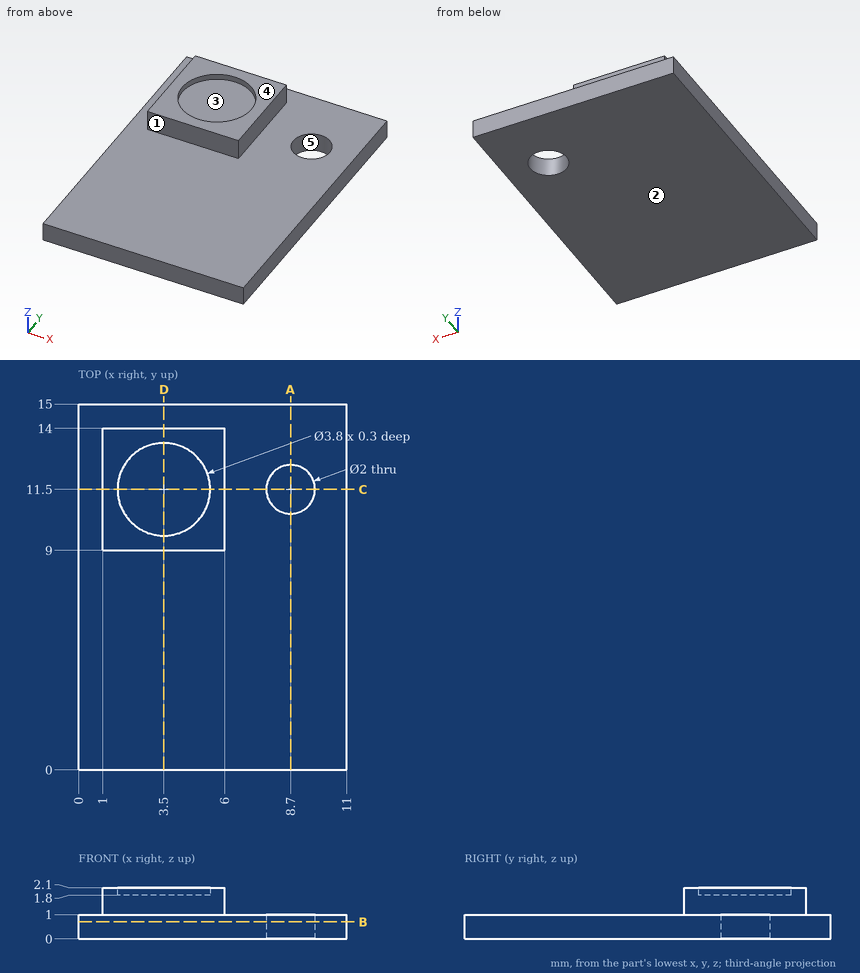
Could you check a few things on this drawing? It's one solid part, dimensions in mm from its lowest x, y, z. A direction names the side the tool comes from. Give positions to 0.01 mm unless a question says otherwise; leave off trailing zeros. Order: outer loops, then holes, each group sorted by start corner. A loop starts at its lowest first (then second) coordinate and runs counter-clockwise, first axis right, second up. Notation, with made-up numbers: M 72,80 L 83,80 A35 cw 83,116 Z; hole C 89.5,-22.75 d11. An arc over 180 degrees is marked long. Use one line per item in the form item = value.
Item 1: Will these pins go through, and if not, where does the flat tip stop? pin 1 Ø3.5 at (x, y) = (3.5, 11.5) entering from +Z; pin 2 Ø2.5 at (x, y) = (8.7, 11.5) entering from +Z; pin 3 Ø0.9 at (y, z) = (11, 1.5) entering from -X.
Values follow:
pin_1 = 1.8
pin_2 = 1
pin_3 = 1
Item 2: If we section it at D-D, the plane x = 3.5: Write out the boundary of the cut face in (y, z), and give its area (3 significant figures).
Values follow:
outline = M 0,0 L 15,0 L 15,1 L 14,1 L 14,2.1 L 13.4,2.1 L 13.4,1.8 L 9.6,1.8 L 9.6,2.1 L 9,2.1 L 9,1 L 0,1 Z
area = 19.4 mm^2
Item 3: If I drill on line 1 along Y through (x, z) = (8.7, 0.3); line 2 along Z through (x, y) = (8, 4); line 3 along Y through (x, z) = (5, 1.1), over which ranges is the centre line in solid material (lowest first)? Write a range as [from, to].
Values follow:
line_1 = [0, 10.5], [12.5, 15]
line_2 = [0, 1]
line_3 = [9, 14]
Item 4: If we section it at A-A, the plane x = 8.7: Write out the boundary of the cut face in (y, z), and give its area (3 significant figures).
Values follow:
outline = M 0,0 L 10.5,0 L 10.5,1 L 0,1 Z; M 12.5,0 L 15,0 L 15,1 L 12.5,1 Z
area = 13.0 mm^2
Item 5: Thinking about a two-plate mould opening in X: for the marked faces 3, 4 and 5, which applies, pulls with the +X half, pulls with the -X half, needs draft (parallel to the pull), parting line crosses it, or undercut?
Values follow:
face_3 = undercut
face_4 = needs draft
face_5 = undercut
Item 6: For the marked faces 1 and 2, which set-ups out of +Z, -Z, +X, -X, +Y, -Y let a thin tool reach every point of the face, with its end or its side?
Values follow:
face_1 = +Z, +X, -X, -Y
face_2 = -Z, +X, -X, +Y, -Y
Item 7: If we section it at C-C, the plane y = 11.5: Write out the boundary of the cut face in (x, z), and give its area (3 significant figures).
Values follow:
outline = M 0,0 L 7.7,0 L 7.7,1 L 6,1 L 6,2.1 L 5.4,2.1 L 5.4,1.8 L 1.6,1.8 L 1.6,2.1 L 1,2.1 L 1,1 L 0,1 Z; M 9.7,0 L 11,0 L 11,1 L 9.7,1 Z
area = 13.4 mm^2
Item 8: If we section it at B-B, the plane z = 0.7: Write out the boundary of the cut face in (x, y).
Values follow:
outline = M 0,0 L 11,0 L 11,15 L 0,15 Z; hole C 8.7,11.5 d2
